Here's the drawing with two shaded views (mm, measured from the low corner). I have some questions. A direction names the side the tool comes from. Give positions to 0.01 mm unless a question says otherwise; leave off trailing zeros. Loops run counter-clockwise (first coordinate to the right, second up) from the corner with the lowest first, then second, coordinate; pieces in that order, holes last. Notation, with made-up numbers: (11, 0.25) -> (61, 0.25) arc R7 ccw to (61, 9.25) -> close; hole circle Ø5 at (-0.5, 87.5). An arc over 180 degrees is marked (long way). Answer in a Markdown table with one row per item. Add a question column.
Item 1: If we section it at D-D (y = 28): Write out the boundary of the cut face in (x, z), then the cut area to 4 significant figures.
Item 2: If we section it at C-C (z = 6): Write out the boundary of the cut face in (x, y).
Item 3: For P1, Ø9, axis at x = 15, y = 15, coming from the -Z side; P2, Ø1.5, axis at x = 8, y = 10, coming from the +Z side; P3, Ø16.5, axis at y = 17.5, z = 25, coming from the -X side; P4, Ø1, axis at x = 10, y = 7, coming from the -Z side, each with a flat end and sliding along its axis, tell me the tip position at first contact or that it passes through.
Item 4: We'd pull the mould along Y, two halves only. Please class the marked faces 1, 2, 3 and 4: released by +Y, released by -Y, zero draft, split by the parting line, or undercut.
Item 5: If I drill on line 1 (Y direction, x = 15, z = 11); line 2 (X direction, y = 10.5, z = 18.5), over which ranges is the centre line in solid material (lowest first)?
Item 6: If we section it at A-A (y = 15): Give the number of separate pieces and of enclosed holes in the cut face, then the cut area to 4 significant figures.
Item 7: If we section it at B-B (x = 15): Write out the boundary of the cut face in (y, z), then the cut area to 3 significant figures.
Item 8: Which directions (+Z, -Z, +X, -X, +Y, -Y) give clear straight access to the entire face, cutting with the end or side of a thin tool? Please do the marked faces 5 and 6.
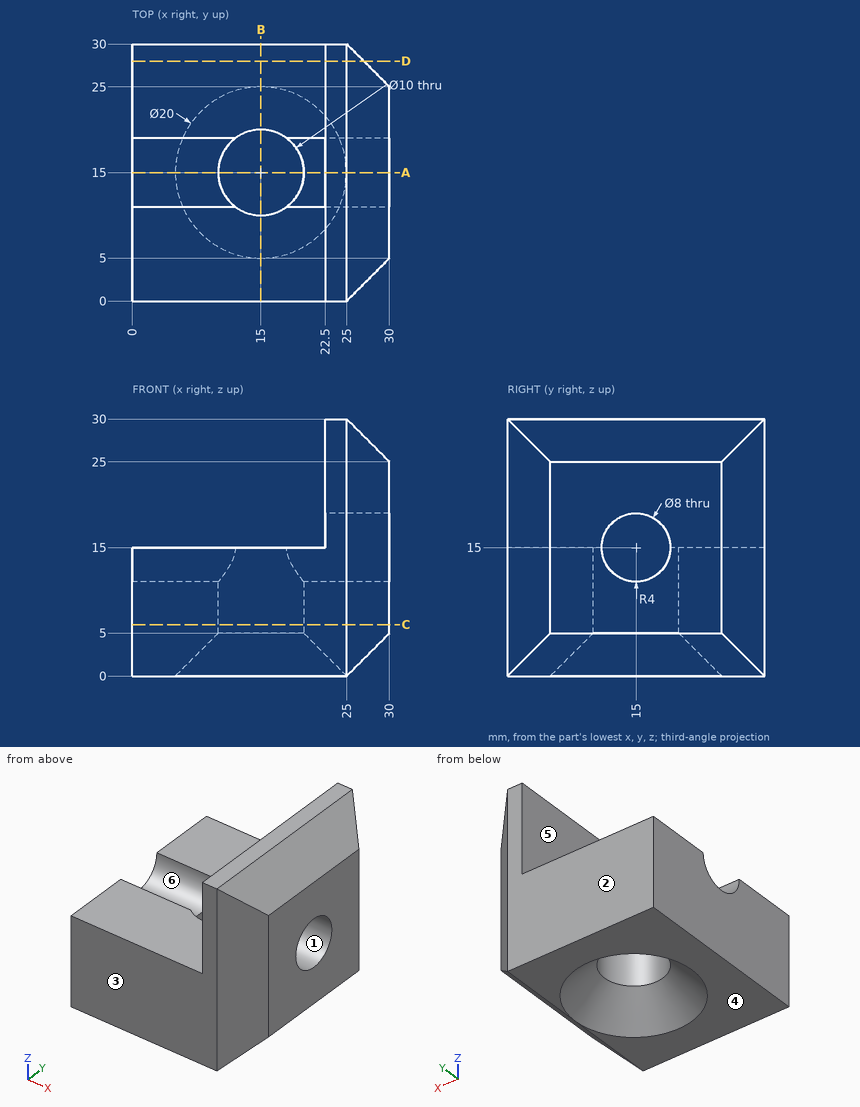
Recorded:
| question | item | result |
|---|---|---|
| 1 | outline | (0, 0) -> (25, 0) -> (27, 2) -> (27, 28) -> (25, 30) -> (22.5, 30) -> (22.5, 15) -> (0, 15) -> close |
| 1 | area | 468.5 mm^2 |
| 2 | outline | (0, 0) -> (25, 0) -> (30, 5) -> (30, 25) -> (25, 30) -> (0, 30) -> close; hole circle Ø10 at (15, 15) |
| 3 | P1 | passes through |
| 3 | P2 | stops at z = 15 |
| 3 | P3 | stops at x = 22.5 |
| 3 | P4 | stops at z = 0.07 |
| 4 | face 1 | undercut |
| 4 | face 2 | released by +Y |
| 4 | face 3 | released by -Y |
| 4 | face 4 | zero draft |
| 5 | line 1 | y = 0 to 10, 20 to 30 |
| 5 | line 2 | x = 22.5 to 30 |
| 6 | separate pieces | 3 |
| 6 | enclosed holes | 0 |
| 6 | area | 252.5 mm^2 |
| 7 | outline | (0, 0) -> (5, 0) -> (10, 5) -> (10, 15) -> (0, 15) -> close; (20, 5) -> (25, 0) -> (30, 0) -> (30, 15) -> (20, 15) -> close |
| 7 | area | 275 mm^2 |
| 8 | face 5 | +Z, -X, +Y, -Y |
| 8 | face 6 | +Z, +X, -X |
